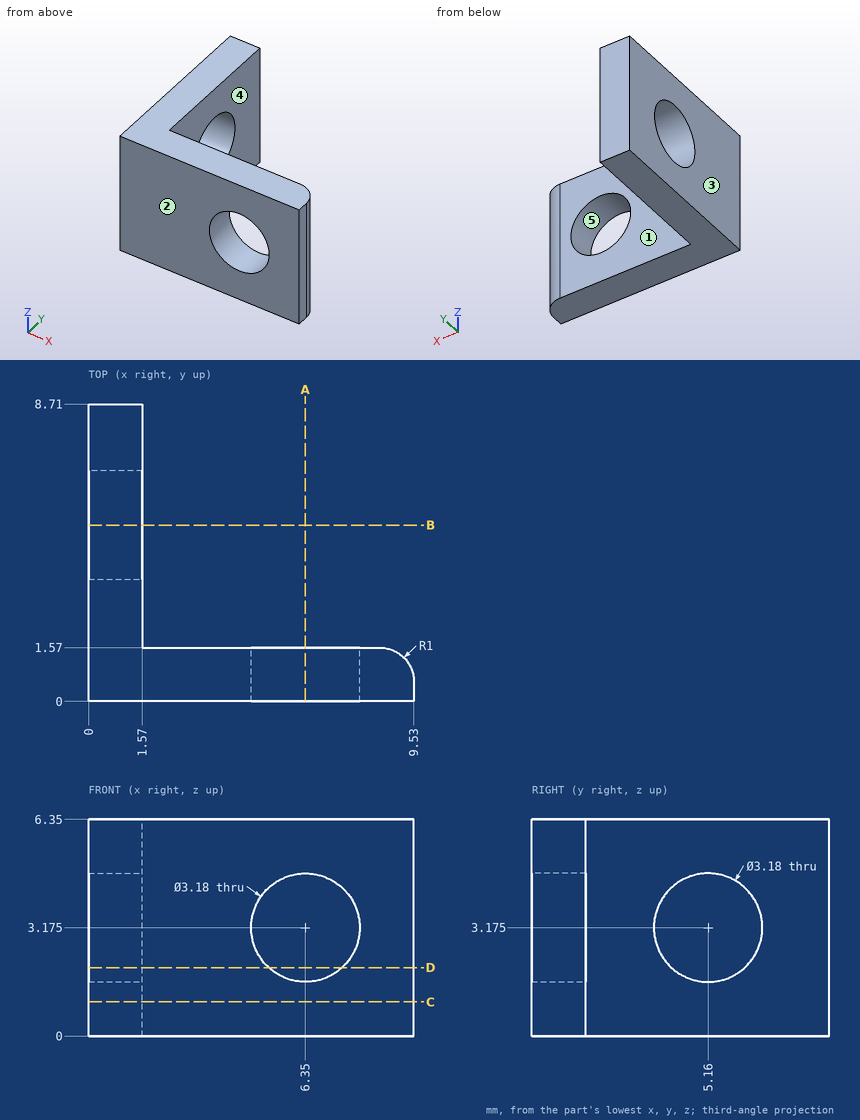
Input: dimensioned drawing with shaded views. Units: mm. Origin: part minimum x, y, z. A direction names the side the tool comes from. Give positions to 0.01 mm unless a question says otherwise; leave off trailing zeros. Write each loop counter-clockwise with the first axis right and the second up, starting at its lowest first coordinate (ties: lowest second). Pieces come first, ordered by that corner, then holes. Notation, with made-up numbers: (34, 64) - (60, 64) arc R17 cw to (60, 76) - close; hole circle Ø1 at (-22, 41.5). An arc over 180 degrees is marked (long way). Write item = value, one per line. Start each with the question number.
1) Material intervals for L1, parallel to Y at x = 1.5, z = 3.25; L2, parallel to Z at x = 1, y = 5.16 (3 decimals); L3, parallel to Y at x = 3, z = 2, sorted ascending. Write a range as [from, to].
2) Cut plane C-C (z = 1). Return loops of the section in (x, y), and give its area (3 significant figures).
3) Cut plane A-A (x = 6.35). Return loops of the section in (y, z) (3 decimals), and give its area (3 significant figures).
4) Cut plane D-D (z = 2). Return loops of the section in (x, y), and give its area (3 significant figures).
5) Draft query along X for the marked faces 3, 4 and 5. Return one class per face: pulls with the +X half, pulls with the -X half, needs draft (parallel to the pull), parting line crosses it, or undercut.
6) Reachability of the marked faces 1 and 2 from +Z, -Z, +X, -X, +Y, -Y: full face, straight path, thin tool, end or side. Return the list, or none.
7) Pin query (flat end, axial travel): pin 1 (2.5 mm diameter, centred on x = 6.35, z = 3.175, fed in from +Y). Return the tip coordinate at first contact, or that it passes through.
Answers follow:
q1.L1 = [0, 3.57], [6.75, 8.71]
q1.L2 = [0, 1.585], [4.765, 6.35]
q1.L3 = [0, 1.57]
q2.outline = (0, 0) - (9.53, 0) - (9.53, 0.57) arc R1 ccw to (8.53, 1.57) - (1.57, 1.57) - (1.57, 8.71) - (0, 8.71) - close
q2.area = 26.0 mm^2
q3.outline = (0, 0) - (1.57, 0) - (1.57, 1.585) - (0, 1.585) - close; (0, 4.765) - (1.57, 4.765) - (1.57, 6.35) - (0, 6.35) - close
q3.area = 4.98 mm^2
q4.outline = (0, 0) - (5.28, 0) - (5.28, 1.57) - (1.57, 1.57) - (1.57, 4.09) - (0, 4.09) - close; (0, 6.23) - (1.57, 6.23) - (1.57, 8.71) - (0, 8.71) - close; (7.42, 0) - (9.53, 0) - (9.53, 0.57) arc R1 ccw to (8.53, 1.57) - (7.42, 1.57) - close
q4.area = 19.2 mm^2
q5.face_3 = pulls with the -X half
q5.face_4 = pulls with the +X half
q5.face_5 = undercut
q6.face_1 = +Z, -Z, +X, +Y
q6.face_2 = +Z, -Z, +X, -X, -Y
q7.pin_1 = through
